Geometry check sheet. Reference: drawing and pictorial views, mm from the part's lowest x, y, z. A direction names the side the tool comes from. Give positions to 0.01 mm unless a question says otherwise; leave off trailing zeros. Order: outer loops, then holes, each group sorted by start corner. A loop starts at its lowest first (then second) coordinate and runs counter-clockwise, first axis right, second up. Notation, with made-up numbers: M -8,24 L 22,24 A26 ccw 22,46 Z; hole C -4,83 d1. An arc over 180 degrees is marked long. Use CSV: the item, a comma, the result in double quotes. Start each with the question number.
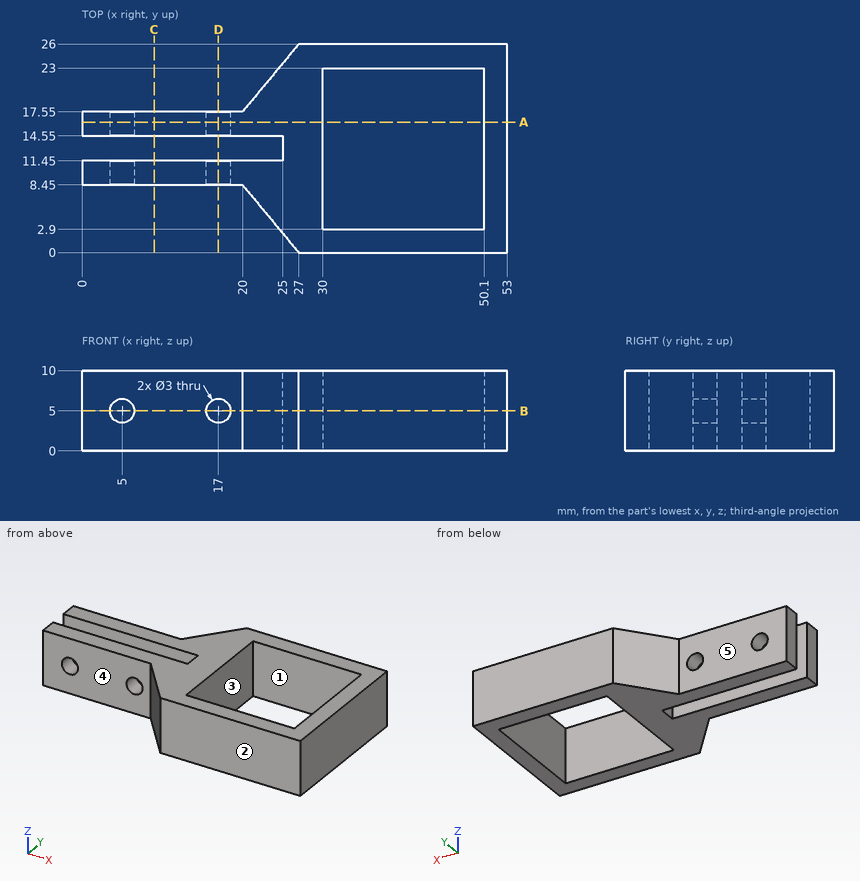
(1) Sectioned sample at B-B on z = 5. Give the number of separate pieces and of enclosed holes in the cut face, then the cut area to 3 significant figures.
(2) Sectioned sample at C-C on x = 9. Record the cut outline in (y, z), then the cut area to 3 significant figures.
(3) Go/stop test with flat-tipped pins: P1, Ø5, axis at x = 17, z = 5, coming from the +Y side; P2, Ø3, axis at x = 10.5, z = 5.5, coming from the -Y side. Record where each tip stops, or that it passes through.
(4) Thickness scan on line 1 (X direction, y = 16.3, z = 5); line 2 (X direction, y = 11.75, z = 5); line 3 (Y direction, x = 8, z = 8.75). Record the ranges inside material, lowest first.
(5) Draft check along Y on the marked faces 3, 4 and 5. Enter one of: +Y half, -Y half, draft (parallel to the pull), parting line (faces both ways), or undercut.
(6) Sectioned sample at A-A on y = 16.25. Record the cut outline in (x, z), then the cut area to 3 significant figures.
(7) Access from +Z, -Z, +X, -X, +Y, -Y to the whole of each face (thin tool, end or side, straight path). Record for the marked faces 1 and 2.
(8) Sectioned sample at D-D on x = 17. Record the cut outline in (y, z), then the cut area to 3 significant figures.
Responses:
1,separate pieces,"5"
1,enclosed holes,"1"
1,area,"463 mm2"
2,outline,"M 8.45,0 L 11.45,0 L 11.45,10 L 8.45,10 Z; M 14.55,0 L 17.55,0 L 17.55,10 L 14.55,10 Z"
2,area,"60.0 mm2"
3,P1,"y = 17.55"
3,P2,"y = 8.45"
4,line 1,"0 to 3.5, 6.5 to 15.5, 18.5 to 30, 50.1 to 53"
4,line 2,"25 to 30, 50.1 to 53"
4,line 3,"8.45 to 11.45, 14.55 to 17.55"
5,face 3,"undercut"
5,face 4,"-Y half"
5,face 5,"+Y half"
6,outline,"M 0,0 L 30,0 L 30,10 L 0,10 Z; M 50.1,0 L 53,0 L 53,10 L 50.1,10 Z; hole C 5,5 d3; hole C 17,5 d3"
6,area,"315 mm2"
7,face 1,"+Z, -Z"
7,face 2,"+Z, -Z, +X, -X, -Y"
8,outline,"M 8.45,0 L 11.45,0 L 11.45,3.5 L 8.45,3.5 Z; M 8.45,6.5 L 11.45,6.5 L 11.45,10 L 8.45,10 Z; M 14.55,0 L 17.55,0 L 17.55,3.5 L 14.55,3.5 Z; M 14.55,6.5 L 17.55,6.5 L 17.55,10 L 14.55,10 Z"
8,area,"42.0 mm2"
